Autodesk Fusion 360 part; units mm, degrees
sketch "Sketch1" plane through (0, 0, 0) normal (0, 0, 1) x (1, 0, 0)
  line L0 (-5.06, 0) -> (-9.94, 0)
  line L1 (-9.94, 0) -> (-9.94, -5.17)
  line L2 (-9.94, -5.17) -> (-5.06, -5.17)
  line L3 (-5.06, -5.17) -> (-5.06, 0)
  line L4 (-9.94, 0) -> (5.06, 0)
  line L5 (5.06, 0) -> (9.94, 0)
  line L6 (9.94, 0) -> (9.94, -5.17)
  line L7 (9.94, -5.17) -> (5.06, -5.17)
  line L8 (5.06, -5.17) -> (5.06, 0)
  line L9 (-5.06, 0) -> (5.06, 0)
  line L10 (5.06, 0) -> (5.06, -0.85)
  line L11 (5.06, -0.85) -> (-5.06, -0.85)
  line L12 (-5.06, -0.85) -> (-5.06, 0)
  circle A0 centre (7.56, -2.7) radius 1.25
  circle A1 centre (-7.44, -2.7) radius 1.25
  line L13 (-7.44, -2.7) -> (-5.06, -2.7) construction
  line L14 (-7.44, -2.7) -> (-7.44, 0) construction
  line L15 (7.56, -2.7) -> (7.56, 0) construction
  line L16 (7.56, -2.7) -> (9.94, -2.7) construction
  dimension "d1" = 4.88
  dimension "d2" = 5.17
  dimension "d4" = 0.85
  dimension "d5" = 2.5
  dimension "d6" = 2.7
  dimension "d7" = 2.5
  dimension "d10" = 15
extrude "Extrude1" add sketch "Sketch1" along normal blind 6
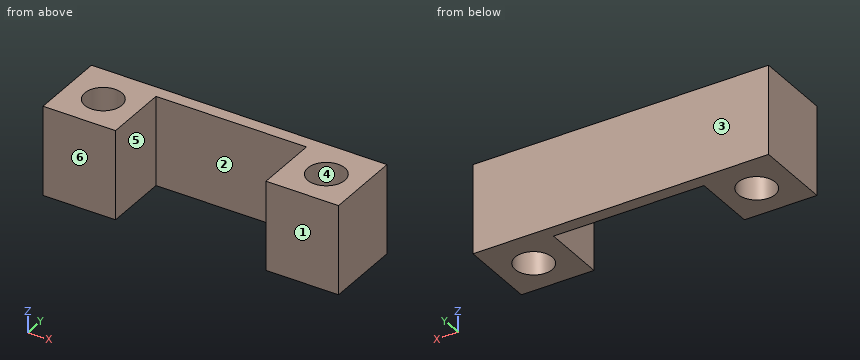
Can you work these out from the model? Positions are in its coordinate system, mm. Face numbers are marked on the shaded views. A direction names the side the tool comes from. Round coordinates to 2 decimals unless told otherwise and drop trailing zeros. Order: outer loops, then holes, each group sorted by start corner. A loop starts at its lowest first (then second) coordinate and runs counter-clockwise, first axis right, second up. Notation, with made-up numbers: M 83.5,32.25 L 102.5,32.25 A24 cw 102.5,71.25 Z; hole C 35,16.5 d8. An arc over 180 degrees is marked long. Use a Markdown table: item, result.
1) If we mould it in two halves opening along Y, with no side actions, what happens to the marked faces 3, 4, 5 and 6? For each: +Y half, -Y half, draft (parallel to the pull), parting line (faces both ways), or undercut.
Geometry says:
| item | result |
|---|---|
| face 3 | +Y half |
| face 4 | undercut |
| face 5 | draft |
| face 6 | -Y half |
2) Imagine slicing it at D-D (y = -4.55). List the corners of the cut face in (x, z) for me, then the cut area to 3 significant figures.
Geometry says:
| item | result |
|---|---|
| outline | M -9.94,0 L -5.06,0 L -5.06,6 L -9.94,6 Z; M 5.06,0 L 9.94,0 L 9.94,6 L 5.06,6 Z |
| area | 58.6 mm² |
3) If I drill on line 1 along X through (y, z) = (-4.15, 1.4); line 2 along Y through (x, z) = (-7.44, 2.95); line 3 along Y through (x, z) = (-3.75, 3.4), over which ranges is the centre line in solid material (lowest first)?
Geometry says:
| item | result |
|---|---|
| line 1 | x = -9.94 to -5.06, 5.06 to 9.94 |
| line 2 | y = -5.17 to -3.95, -1.45 to 0 |
| line 3 | y = -0.85 to 0 |
4) On a 3-axis mill with a long thin cutter (end or side, diameter ignored), from which of +Z, -Z, +X, -X, +Y, -Y can I reach the whole of each face in a straight line? I mean the marked faces 1 and 2. Say none if no direction works.
Geometry says:
| item | result |
|---|---|
| face 1 | +Z, -Z, +X, -X, -Y |
| face 2 | +Z, -Z, -Y |
5) I'm going to push a flat-ended pin straight in: P1, Ø1.5, axis at x = 0, z = 2.5, coming from the +Y side. Where does the tip first touch, or does it pass through?
Geometry says:
| item | result |
|---|---|
| P1 | stops at y = 0 |
6) Imagine slicing it at B-B (z = 1.8). List the corners of the cut face in (x, y) for me, then the cut area to 3 significant figures.
Geometry says:
| item | result |
|---|---|
| outline | M -9.94,-5.17 L -5.06,-5.17 L -5.06,-0.85 L 5.06,-0.85 L 5.06,-5.17 L 9.94,-5.17 L 9.94,0 L -9.94,0 Z; hole C -7.44,-2.7 d2.5; hole C 7.56,-2.7 d2.5 |
| area | 49.2 mm² |
7) Imagine slicing it at A-A (x = 8). List the corners of the cut face in (y, z) for me, then the cut area to 3 significant figures.
Geometry says:
| item | result |
|---|---|
| outline | M -5.17,0 L -3.87,0 L -3.87,6 L -5.17,6 Z; M -1.53,0 L 0,0 L 0,6 L -1.53,6 Z |
| area | 17.0 mm² |
8) Imagine slicing it at C-C (y = -2.7). List the corners of the cut face in (x, z) for me.
Geometry says:
| item | result |
|---|---|
| outline | M -9.94,0 L -8.69,0 L -8.69,6 L -9.94,6 Z; M -6.19,0 L -5.06,0 L -5.06,6 L -6.19,6 Z; M 5.06,0 L 6.31,0 L 6.31,6 L 5.06,6 Z; M 8.81,0 L 9.94,0 L 9.94,6 L 8.81,6 Z |
